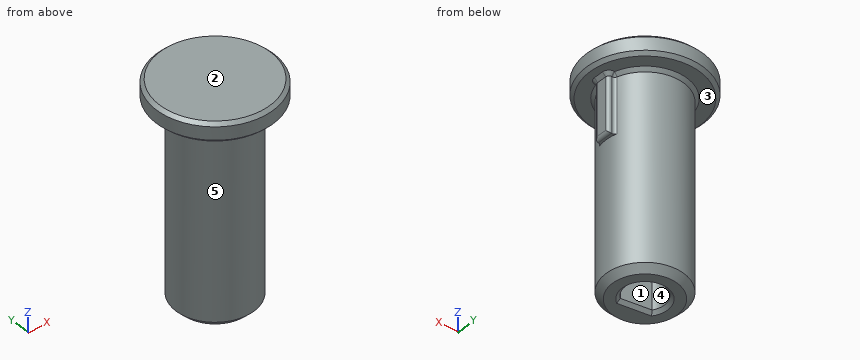
from build123d import *

# Parameters (mm, degrees)
SKETCH1_R           = 9
BOSS_EXTRUDE1_DEPTH = 3
SKETCH2_R           = 6
BOSS_EXTRUDE2_DEPTH = 30
SKETCH3_W           = 1.649682621
SKETCH3_H           = 2.5
BOSS_EXTRUDE3_DEPTH = 9
FILLET1_R           = 0.5
CHAMFER1_SIZE       = 0.5
CHAMFER2_SIZE       = 1
CUT_EXTRUDE1_DEPTH  = 10
CHAMFER3_SIZE       = 0.5


with BuildPart() as part:
    # Sketch1 → Boss-Extrude1 (new body)
    with BuildSketch(Plane.XY):
        Circle(SKETCH1_R)
    extrude(amount=BOSS_EXTRUDE1_DEPTH)

    # Sketch2 → Boss-Extrude2 (add)
    with BuildSketch(Plane(origin=(0, 0, 0), x_dir=(-1, 0, 0), z_dir=(0, 0, -1))):
        Circle(SKETCH2_R)
    extrude(amount=BOSS_EXTRUDE2_DEPTH)

    # Sketch3 → Boss-Extrude3 (add)
    with BuildSketch(Plane(origin=(0, 0, 0), x_dir=(-1, 0, 0), z_dir=(0, 0, -1))):
        with Locations((-5.999366701, 0.087173351)):
            Rectangle(SKETCH3_W, SKETCH3_H)
    extrude(amount=BOSS_EXTRUDE3_DEPTH)

    # Fillet1
    fillet1_edges = [part.edges().sort_by_distance(p)[0] for p in [
        (5.849099711, 1.337173351, -4.5),
        (5.886241091, -1.162826649, -4.5),
        (6.824208011, -1.162826649, -4.5),
        (6.824208011, 1.337173351, -4.5),
        (6.824208011, 0.087173351, -9),
    ]]
    fillet(fillet1_edges, radius=FILLET1_R)

    # Chamfer1
    chamfer1_edges = [part.edges().sort_by_distance(p)[0] for p in [
        (-9, 0, 0),
        (6.303958853, -1.162826649, 0),
        (-0.773923618, -5.949877497, 0),
        (6.824208011, 0.087173351, 0),
        (6.279586727, 1.337173351, 0),
        (5.935516377, 1.436760743, 0),
        (5.978713688, -1.266622868, 0),
        (6.677761402, -1.016380039, 0),
        (6.677761402, 1.190726742, 0),
        (-9, 0, 3),
    ]]
    chamfer(chamfer1_edges, length=CHAMFER1_SIZE - 0.0001)  # a hair under: the kernel refuses the full size

    # Chamfer2
    chamfer2_edges = [part.edges().sort_by_distance(p)[0] for p in [
        (6, 0, -30),
    ]]
    chamfer(chamfer2_edges, length=CHAMFER2_SIZE)

    # Sketch4 → Cut-Extrude1 (cut)
    with BuildSketch(Plane(origin=(0, 0, -30), x_dir=(-1, 0, 0), z_dir=(0, 0, -1))):
        with BuildLine():
            Line((-1.922298895, -2.303207971), (2.50253525, -1.654484005))
            ThreePointArc((2.50253525, -1.654484005), (-0.435177266, 2.968268982), (-1.922298895, -2.303207971))
        make_face()
    extrude(amount=-CUT_EXTRUDE1_DEPTH, mode=Mode.SUBTRACT)

    # Chamfer3
    chamfer3_edges = [part.edges().sort_by_distance(p)[0] for p in [
        (0.435177266, 2.968268982, -30),
        (-0.290118177, -1.978845988, -30),
    ]]
    chamfer(chamfer3_edges, length=CHAMFER3_SIZE)


solid = part.part
The listing builds one solid part. Answer for the finished solid, in the listing's coordinates (mm). Face numbers are marked on the shaded views. A direction names the side the tool comes from. Give positions to 0.01 mm unless a question says otherwise; leave off trailing zeros. Write each loop counter-clockwise with the first axis right and the second up, starting at its lowest first coordinate (ties: lowest second). Pieces come first, ordered by that corner, then holes. Notation, with made-up numbers: (-4, 51) - (42, 51) arc R7 ccw to (42, 64) - close; hole circle Ø7 at (0, 43.5). An arc over 180 degrees is marked (long way). One line per question, with ' | ' between items. Start each with the question number.
1. Straight lines are drawn through the part: line 1 (X direction, y = 0, z = -26); line 2 (Z direction, x = 2.25, y = 6.75); line 3 (Y direction, x = 0, z = -22.5). For each, find the intervals that lie inside material, in ascending order.
2. For the marked faces 1 and 2, determine the directions among +Z, -Z, +X, -X, +Y, -Y from which every point of the face is accessible in a straight line to the end or side of a thin tool.
3. Determine the mould class of the marked faces 3, 4 and 5 for opening direction Y: +Y half, -Y half, draft (parallel to the pull), parting line (faces both ways), or undercut.
4. Given P1, Ø1, axis at y = -4, z = -26.5, coming from the +X side; P2, Ø5, axis at y = -1, z = -21, coming from the -X side; P3, Ø3, axis at y = 0.5, z = -16.5, coming from the +X side, each flat-ended and moving along its own axis, determine where each tip first touches the part or whether it passes through.
5. Section B-B, the plane x = 0 is taken. Determine the outline of the cut face in (y, z), then the cut area to 3 significant figures.
6. Section A-A, the plane y = 0 is taken. Determine the outline of the cut face in (x, z).
Result:
1) line 1: x = -6 to -3, 3 to 6 | line 2: z = 0 to 3 | line 3: y = -6 to -2.02, 3 to 6
2) face 1: -Z | face 2: +Z, +X, -X, +Y, -Y
3) face 3: draft | face 4: undercut | face 5: parting line
4) P1: stops at x = 4.87 | P2: stops at x = -6 | P3: stops at x = 6
5) outline: (-9, 0.5) - (-8.5, 0) - (-6.5, 0) - (-6, -0.5) - (-6, -29) - (-5, -30) - (-2.53, -30) - (-2.02, -29.5) - (-2.02, -20) - (3, -20) - (3, -29.5) - (3.5, -30) - (5, -30) - (6, -29) - (6, -0.5) - (6.5, 0) - (8.5, 0) - (9, 0.5) - (9, 2.5) - (8.5, 3) - (-8.5, 3) - (-9, 2.5) - close | area: 362 mm2
6) outline: (-9, 0.5) - (-8.5, 0) - (-6.5, 0) - (-6, -0.5) - (-6, -29) - (-5, -30) - (-3.5, -30) - (-3, -29.5) - (-3, -20) - (3, -20) - (3, -29.5) - (3.5, -30) - (5, -30) - (6, -29) - (6, -9) - (6.32, -9) arc R0.5 ccw to (6.82, -8.5) - (6.82, -0.5) - (7.32, 0) - (8.5, 0) - (9, 0.5) - (9, 2.5) - (8.5, 3) - (-8.5, 3) - (-9, 2.5) - close
